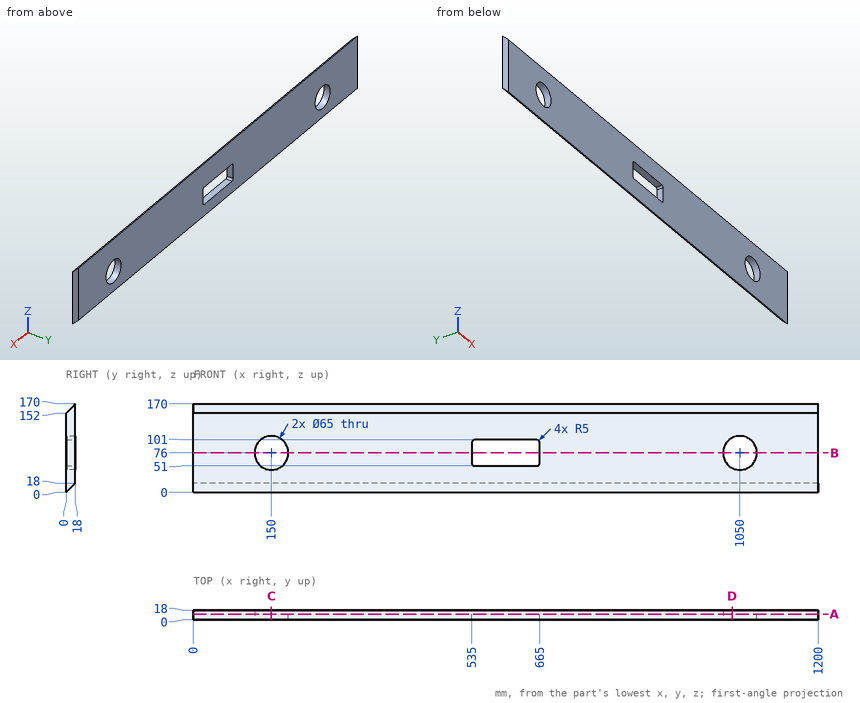
Answer from the drawing. Dimensions are ordinates in mm from the lowest x, y and z of the part. Give positions to 0.01 mm unless a question says otherwise; leave off trailing zeros. Loops run counter-clockwise (first coordinate to the right, second up) from the corner with the lowest first, then second, coordinate; pieces in that order, holes last.
Item 1: The part is cut by section D-D (x = 1035). Write down the section's boundary in (y, z).
Item 2: The part is cut by section B-B (z = 76). Write down the section's boundary in (x, y), and give its area (3 significant figures).
Item 3: The part is cut by section C-C (x = 150). Write down the section's boundary in (y, z), and give its area (3 significant figures).
Item 4: Each of these flat-tipped pins is pushed along its axis until it touches: pin 1 Ø3 at (x, y) = (362.5, 11.5) entering from -Z; pin 2 Ø5.5 at (x, y) = (573, 4.5) entering from -Z; pin 3 Ø5.5 at (x, y) = (594.5, 9) entering from +Z. Where does it stop, or does it pass through?
Item 5: The part is cut by section A-A (y = 11). Write down the section's boundary in (x, z), and give its area (3 significant figures).
Item 6: Find the intervals of material crossed by line 1 along X through (y, z) = (12.5, 82.5); line 2 along X through (y, z) = (7.5, 85.5); line 3 along X through (y, z) = (17.25, 47), in increasing order.
Taken from the geometry:
1. outline: (0, 0) - (18, 18) - (18, 47.17) - (0, 47.17) - close; (0, 104.83) - (18, 104.83) - (18, 170) - (0, 152) - close
2. outline: (0, 0) - (117.5, 0) - (117.5, 18) - (0, 18) - close; (182.5, 0) - (535, 0) - (535, 18) - (182.5, 18) - close; (665, 0) - (1017.5, 0) - (1017.5, 18) - (665, 18) - close; (1082.5, 0) - (1200, 0) - (1200, 18) - (1082.5, 18) - close
2. area: 16,900 mm2
3. outline: (0, 0) - (18, 18) - (18, 43.5) - (0, 43.5) - close; (0, 108.5) - (18, 108.5) - (18, 170) - (0, 152) - close
3. area: 1,570 mm2
4. pin 1: stops at z = 10
4. pin 2: stops at z = 1.75
4. pin 3: stops at z = 163.75
5. outline: (0, 11) - (1200, 11) - (1200, 163) - (0, 163) - close; hole circle Ø65 at (150, 76); hole (535, 56) arc R5 ccw to (540, 51) - (660, 51) arc R5 ccw to (665, 56) - (665, 96) arc R5 ccw to (660, 101) - (540, 101) arc R5 ccw to (535, 96) - close; hole circle Ø65 at (1050, 76)
5. area: 169,000 mm2
6. line 1: x = 0 to 118.16, 181.84 to 535, 665 to 1018.16, 1081.84 to 1200
6. line 2: x = 0 to 118.92, 181.08 to 535, 665 to 1018.92, 1081.08 to 1200
6. line 3: x = 0 to 135.33, 164.67 to 1035.33, 1064.67 to 1200
